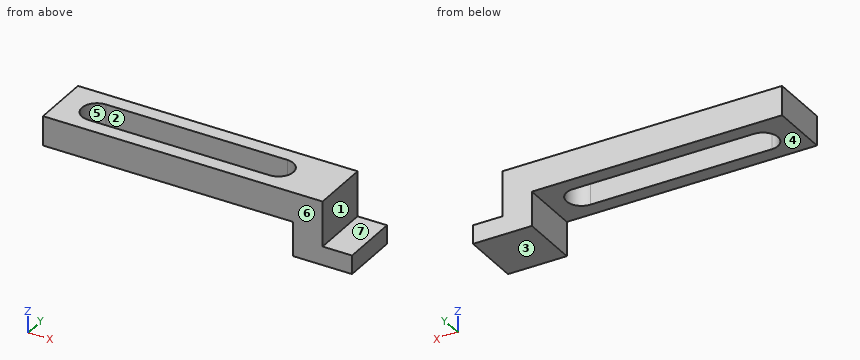
from build123d import *

# Parameters (mm, degrees)
SKETCH_W     = 57
SKETCH_H     = 12
PAD_DEPTH    = 6
BOX_W        = 12
BOX_H        = 12
BOX_DEPTH    = 7
BOX001_W     = 12
BOX001_H     = 6
BOX001_DEPTH = 3.2


with BuildPart() as part:
    # Sketch → Pad (new body)
    with BuildSketch(Plane.XY):
        with Locations((28.5, 6)):
            Rectangle(SKETCH_W, SKETCH_H)
        with BuildLine():
            Line((44.436229, 9.05), (7.436229, 9.05))
            ThreePointArc((7.436229, 9.05), (4.386229, 6), (7.436229, 2.95))
            Line((7.436229, 2.95), (44.436229, 2.95))
            ThreePointArc((44.436229, 2.95), (47.486229, 6), (44.436229, 9.05))
        make_face(mode=Mode.SUBTRACT)
    extrude(amount=PAD_DEPTH)

    # Box → Box (join)
    with BuildSketch(Plane(origin=(51, 0, 0), x_dir=(0, 1, 0), z_dir=(0, 0, -1))):
        with Locations((6, 6)):
            Rectangle(BOX_W, BOX_H)
    extrude(amount=BOX_DEPTH)

    # Box001 → Box001 (cut)
    with BuildSketch(Plane(origin=(57, 0, 0), x_dir=(0, 1, 0), z_dir=(0, 0, -1))):
        with Locations((6, 3)):
            Rectangle(BOX001_W, BOX001_H)
    extrude(amount=BOX001_DEPTH, mode=Mode.SUBTRACT)


solid = part.part
Can you work these out from the model? Positions are in its coordinate system, mm. Face numbers are marked on the shaded views. A direction names the side the tool comes from. Round coordinates to 2 decimals unless told otherwise and drop trailing zeros. Order: outer loops, then holes, each group sorted by start corner. A loop starts at its lowest first (then second) coordinate and runs counter-clockwise, first axis right, second up. Notation, with made-up numbers: M 59.5,59.25 L 103.5,59.25 A32 cw 103.5,93.25 Z; hole C -15.5,32.25 d2. An arc over 180 degrees is marked long. Use a Markdown table: item, result.
1) Imagine slicing it at B-B (y = 6). List the corners of the cut face in (x, z) for me, then the cut area to 3 significant figures.
Geometry says:
| item | result |
|---|---|
| outline | M 0,0 L 4.39,0 L 4.39,6 L 0,6 Z; M 47.49,0 L 51,0 L 51,-7 L 63,-7 L 63,-3.2 L 57,-3.2 L 57,6 L 47.49,6 Z |
| area | 148 mm² |
2) Imagine slicing it at A-A (x = 33). List the corners of the cut face in (y, z) for me.
Geometry says:
| item | result |
|---|---|
| outline | M 0,0 L 2.95,0 L 2.95,6 L 0,6 Z; M 9.05,0 L 12,0 L 12,6 L 9.05,6 Z |
3) If we mould it in two halves opening along X, with no side actions, what happens to the marked faces 1, 2 and 3? For each: +X half, -X half, draft (parallel to the pull), parting line (faces both ways), or undercut.
Geometry says:
| item | result |
|---|---|
| face 1 | +X half |
| face 2 | undercut |
| face 3 | draft |
4) Imagine slicing it at C-C (z = 3.5). List the corners of the cut face in (x, y) for me, then the cut area to 3 significant figures.
Geometry says:
| item | result |
|---|---|
| outline | M 0,0 L 57,0 L 57,12 L 0,12 Z; hole M 7.44,2.95 L 44.44,2.95 A3.05 ccw 44.44,9.05 L 7.44,9.05 A3.05 ccw Z |
| area | 429 mm² |
5) I'm going to push flat-ended pins straight in: P1, Ø6, axis at y = 3, z = 0, coming from the +X side; P2, Ø6, axis at x = 35, y = 8, coming from the -Z side; P3, Ø5.5, axis at y = 4, z = -5, coming from the -X side. Where does each tip first touch, or does it pass through?
Geometry says:
| item | result |
|---|---|
| P1 | stops at x = 57 |
| P2 | stops at z = 0 |
| P3 | stops at x = 51 |
6) On a 3-axis mill with a long thin cutter (end or side, diameter ignored), from which of +Z, -Z, +X, -X, +Y, -Y can I reach the whole of each face in a straight line? I mean the marked faces 4, 5, 6 and 7. Say none if no direction works.
Geometry says:
| item | result |
|---|---|
| face 4 | -Z, -X, +Y, -Y |
| face 5 | +Z, -Z |
| face 6 | +Z, -Z, +X, -X, -Y |
| face 7 | +Z, +X, +Y, -Y |
7) If I drill on line 1 along Y through (x, z) = (12, 4.5); line 2 along Z through (x, y) = (59, 5), over which ranges is the centre line in solid material (lowest first)?
Geometry says:
| item | result |
|---|---|
| line 1 | y = 0 to 2.95, 9.05 to 12 |
| line 2 | z = -7 to -3.2 |
8) Imagine slicing it at D-D (x = 46.5). List the corners of the cut face in (y, z) for me.
Geometry says:
| item | result |
|---|---|
| outline | M 0,0 L 3.75,0 L 3.75,6 L 0,6 Z; M 8.25,0 L 12,0 L 12,6 L 8.25,6 Z |
